Source: three-view drawing plus pictorial views. Frame: mm from the lowest corner of the part. Coordinates: 2 decimals unless noted, no trailing zeros. Loops run counter-clockwise (first coordinate to the right, second up) from the corner with the lowest first, then second, coordinate; pieces in that order, holes last. Notation, with made-up numbers: M 54,32.25 L 58,32.25 A21 ccw 58,42.25 Z; hole C 6.25,-11 d5. An arc over 180 degrees is marked long. Use a Markdown table: item, result. Add a question column.
1. Line query: L1, parallel to Y at x = 60, z = 21; L2, parallel to Z at x = 44, y = 71; L3, parallel to Y at x = 60, z = 46. Output: solid intervals per line, ascending. Write a range as [from, to].
2. Draft query along X for the marked faces 1, 2 and 3. Return one class per face: +X half, -X half, draft (parallel to the pull), parting line (faces both ways), or undercut.
3. Section A-A on z = 27. Output: boundary loops of the cut face in (x, y).
4. Pin query (flat end, axial travel): pin 1 (21 mm diameter, centred on x = 64.5, y = 67.5, fed in from +Z); pin 2 (2 mm diameter, centred on x = 86.5, z = 28, fed in from -Y); pin 3 (5 mm diameter, centred on y = 69.5, z = 18, fed in from +X). Return the tip coordinate at first contact, or that it passes through.
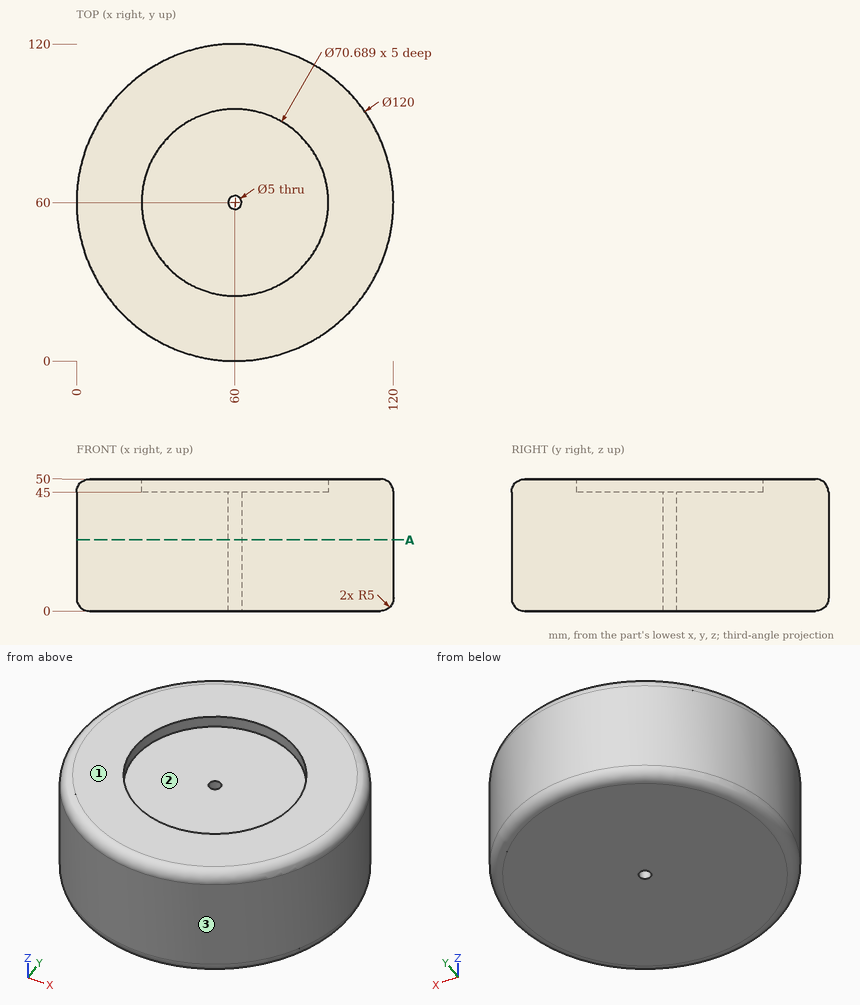
Answers below:
| question | item | result |
|---|---|---|
| 1 | L1 | y = [0, 57.5], [62.5, 120] |
| 1 | L2 | z = [0, 45] |
| 1 | L3 | y = [0.1, 24.66], [95.34, 119.9] |
| 2 | face 1 | draft |
| 2 | face 2 | undercut |
| 2 | face 3 | parting line |
| 3 | outline | C 60,60 d120; hole C 60,60 d5 |
| 4 | pin 1 | stops at z = 45 |
| 4 | pin 2 | stops at y = 5.69 |
| 4 | pin 3 | stops at x = 119.59 |
